```python
from build123d import *

# Parameters (mm, degrees)
SKETCH_W           = 37
SKETCH_H           = 51.5
PAD_DEPTH          = 25
SKETCH001_W        = 31
SKETCH001_H        = 45.5
POCKET_DEPTH       = 22
SKETCH002_W        = 31.0000008352
SKETCH002_H        = 3
POCKET001_DEPTH    = 22
SKETCH003_R        = 2
POCKET002_DEPTH    = 5
SKETCH004_R        = 3
POCKET003_DEPTH    = 1
SKETCH005_W        = 4
SKETCH005_H        = 3
PAD001_DEPTH       = 22
PAD001_FACE12_W    = 45.5
PAD001_FACE12_H    = 22
POCKET004_DEPTH    = 0.1
POCKET004_FACE17_W = 3.9999991648
POCKET004_FACE17_H = 22
POCKET005_DEPTH    = 0.1
POCKET005_FACE13_W = 31
POCKET005_FACE13_H = 22
POCKET006_DEPTH    = 0.1
POCKET006_FACE12_W = 45.5
POCKET006_FACE12_H = 22
POCKET007_DEPTH    = 0.1
POCKET007_FACE11_W = 4
POCKET007_FACE11_H = 22
POCKET008_DEPTH    = 0.1
POCKET008_FACE19_W = 0.1
POCKET008_FACE19_H = 22
POCKET009_DEPTH    = 0.1
POCKET009_FACE15_W = 0.1
POCKET009_FACE15_H = 22
POCKET010_DEPTH    = 0.1
POCKET010_FACE12_W = 0.1
POCKET010_FACE12_H = 22
POCKET011_DEPTH    = 0.1
POCKET011_FACE22_W = 0.1
POCKET011_FACE22_H = 22
POCKET012_DEPTH    = 0.1
POCKET012_FACE22_W = 45.7
POCKET012_FACE22_H = 22
POCKET013_DEPTH    = 1
POCKET013_FACE12_W = 45.7
POCKET013_FACE12_H = 22
POCKET014_DEPTH    = 1
POCKET014_FACE22_W = 33.2
POCKET014_FACE22_H = 22
POCKET015_DEPTH    = 1
POCKET015_FACE17_W = 5.0999991648
POCKET015_FACE17_H = 22
POCKET016_DEPTH    = 1
POCKET016_FACE11_W = 5.1
POCKET016_FACE11_H = 22
POCKET017_DEPTH    = 1
POCKET017_FACE3_W  = 51.5
POCKET017_FACE3_H  = 25
PAD002_DEPTH       = 1
PAD002_FACE2_W     = 51.5
PAD002_FACE2_H     = 25
PAD003_DEPTH       = 1
PAD003_FACE2_W     = 39
PAD003_FACE2_H     = 25
PAD004_DEPTH       = 1
PAD005_DEPTH       = 1
PAD006_DEPTH       = 5
PAD007_DEPTH       = 3
SKETCH006_W        = 22.9999991648
SKETCH006_H        = 3
PAD008_DEPTH       = 10


with BuildPart() as part:
    # Sketch → Pad (new body)
    with BuildSketch(Plane.XY):
        with Locations((-15.7498351648, -0.8188517965)):
            Rectangle(SKETCH_W, SKETCH_H)
    extrude(amount=PAD_DEPTH)

    # Sketch001 (on Face6 of Pad) → Pocket (cut)
    with BuildSketch(Plane.XY.offset(25)):
        with Locations((-15.7498351648, -0.8188517965)):
            Rectangle(SKETCH001_W, SKETCH001_H)
    extrude(amount=-POCKET_DEPTH, mode=Mode.SUBTRACT)

    # Sketch002 (on Face5 of Pocket) → Pocket001 (cut)
    with BuildSketch(Plane.XY.offset(25)):
        with Locations((-15.7498355824, -25.0688517965)):
            Rectangle(SKETCH002_W, SKETCH002_H)
    extrude(amount=-POCKET001_DEPTH, mode=Mode.SUBTRACT)

    # Sketch003 (on Face12 of Pocket001) → Pocket002 (cut)
    with BuildSketch(Plane.XY.offset(3)):
        with Locations((-15.5998351648, 16.2811482035)):
            Circle(SKETCH003_R)
        with Locations((-27.1998351648, -19.5188517965)):
            Circle(SKETCH003_R)
        with Locations((-4.2998351648, -19.5188517965)):
            Circle(SKETCH003_R)
    extrude(amount=-POCKET002_DEPTH, mode=Mode.SUBTRACT)

    # Sketch004 (on Face4 of Pocket002) → Pocket003 (cut)
    with BuildSketch(Plane(origin=(0, 0, 0), x_dir=(1, 0, 0), z_dir=(0, 0, -1))):
        with Locations((-27.199835, 19.518852)):
            Circle(SKETCH004_R)
        with Locations((-4.29979, 19.518393)):
            Circle(SKETCH004_R)
        with Locations((-15.599835, -16.281149)):
            Circle(SKETCH004_R)
    extrude(amount=-POCKET003_DEPTH, mode=Mode.SUBTRACT)

    # Sketch005 (on Face15 of Pocket003) → Pad001 (join)
    with BuildSketch(Plane.XY.offset(3)):
        with Locations((-29.249836, -25.0688517965)):
            Rectangle(SKETCH005_W, SKETCH005_H)
        with Locations((-2.2498351648, -25.0688517965)):
            Rectangle(SKETCH005_W, SKETCH005_H)
    extrude(amount=PAD001_DEPTH)

    # Pad001 Face12 → Pocket004 (cut)
    with BuildSketch(Plane(origin=(-31.2498351648, -0.8188517965, 14), x_dir=(0, -1, 0), z_dir=(1, 0, 0))):
        Rectangle(PAD001_FACE12_W, PAD001_FACE12_H)
    extrude(amount=-POCKET004_DEPTH, mode=Mode.SUBTRACT)

    # Pocket004 Face17 → Pocket005 (cut)
    with BuildSketch(Plane(origin=(-29.2498355824, -23.5688517965, 14), x_dir=(1, 0, 0), z_dir=(0, 1, 0))):
        Rectangle(POCKET004_FACE17_W, POCKET004_FACE17_H)
    extrude(amount=-POCKET005_DEPTH, mode=Mode.SUBTRACT)

    # Pocket005 Face13 → Pocket006 (cut)
    with BuildSketch(Plane(origin=(-15.7498351648, 21.9311482035, 14), x_dir=(-1, 0, 0), z_dir=(0, -1, 0))):
        Rectangle(POCKET005_FACE13_W, POCKET005_FACE13_H)
    extrude(amount=-POCKET006_DEPTH, mode=Mode.SUBTRACT)

    # Pocket006 Face12 → Pocket007 (cut)
    with BuildSketch(Plane(origin=(-0.2498351648, -0.8188517965, 14), x_dir=(0, 1, 0), z_dir=(-1, 0, 0))):
        Rectangle(POCKET006_FACE12_W, POCKET006_FACE12_H)
    extrude(amount=-POCKET007_DEPTH, mode=Mode.SUBTRACT)

    # Pocket007 Face11 → Pocket008 (cut)
    with BuildSketch(Plane(origin=(-2.2498351648, -23.5688517965, 14), x_dir=(1, 0, 0), z_dir=(0, 1, 0))):
        Rectangle(POCKET007_FACE11_W, POCKET007_FACE11_H)
    extrude(amount=-POCKET008_DEPTH, mode=Mode.SUBTRACT)

    # Pocket008 Face19 → Pocket009 (cut)
    with BuildSketch(Plane(origin=(-31.2998351648, 21.9311482035, 14), x_dir=(-1, 0, 0), z_dir=(0, -1, 0))):
        Rectangle(POCKET008_FACE19_W, POCKET008_FACE19_H)
    extrude(amount=-POCKET009_DEPTH, mode=Mode.SUBTRACT)

    # Pocket009 Face15 → Pocket010 (cut)
    with BuildSketch(Plane(origin=(-0.1998351648, 21.9311482035, 14), x_dir=(-1, 0, 0), z_dir=(0, -1, 0))):
        Rectangle(POCKET009_FACE15_W, POCKET009_FACE15_H)
    extrude(amount=-POCKET010_DEPTH, mode=Mode.SUBTRACT)

    # Pocket010 Face12 → Pocket011 (cut)
    with BuildSketch(Plane(origin=(-0.2498351648, -23.6188517965, 14), x_dir=(0, 1, 0), z_dir=(-1, 0, 0))):
        Rectangle(POCKET010_FACE12_W, POCKET010_FACE12_H)
    extrude(amount=-POCKET011_DEPTH, mode=Mode.SUBTRACT)

    # Pocket011 Face22 → Pocket012 (cut)
    with BuildSketch(Plane(origin=(-31.2498351648, -23.6188517965, 14), x_dir=(0, -1, 0), z_dir=(1, 0, 0))):
        Rectangle(POCKET011_FACE22_W, POCKET011_FACE22_H)
    extrude(amount=-POCKET012_DEPTH, mode=Mode.SUBTRACT)

    # Pocket012 Face22 → Pocket013 (cut)
    with BuildSketch(Plane(origin=(-31.3498351648, -0.8188517965, 14), x_dir=(0, -1, 0), z_dir=(1, 0, 0))):
        Rectangle(POCKET012_FACE22_W, POCKET012_FACE22_H)
    extrude(amount=-POCKET013_DEPTH, mode=Mode.SUBTRACT)

    # Pocket013 Face12 → Pocket014 (cut)
    with BuildSketch(Plane(origin=(-0.1498351648, -0.8188517965, 14), x_dir=(0, 1, 0), z_dir=(-1, 0, 0))):
        Rectangle(POCKET013_FACE12_W, POCKET013_FACE12_H)
    extrude(amount=-POCKET014_DEPTH, mode=Mode.SUBTRACT)

    # Pocket014 Face22 → Pocket015 (cut)
    with BuildSketch(Plane(origin=(-15.7498351648, 22.0311482035, 14), x_dir=(-1, 0, 0), z_dir=(0, -1, 0))):
        Rectangle(POCKET014_FACE22_W, POCKET014_FACE22_H)
    extrude(amount=-POCKET015_DEPTH, mode=Mode.SUBTRACT)

    # Pocket015 Face17 → Pocket016 (cut)
    with BuildSketch(Plane(origin=(-29.7998355824, -23.6688517965, 14), x_dir=(1, 0, 0), z_dir=(0, 1, 0))):
        Rectangle(POCKET015_FACE17_W, POCKET015_FACE17_H)
    extrude(amount=-POCKET016_DEPTH, mode=Mode.SUBTRACT)

    # Pocket016 Face11 → Pocket017 (cut)
    with BuildSketch(Plane(origin=(-1.6998351648, -23.6688517965, 14), x_dir=(1, 0, 0), z_dir=(0, 1, 0))):
        Rectangle(POCKET016_FACE11_W, POCKET016_FACE11_H)
    extrude(amount=-POCKET017_DEPTH, mode=Mode.SUBTRACT)

    # Pocket017 Face3 → Pad002 (add)
    with BuildSketch(Plane(origin=(2.7501648352, -0.8188517965, 12.5), x_dir=(0, -1, 0), z_dir=(1, 0, 0))):
        Rectangle(POCKET017_FACE3_W, POCKET017_FACE3_H)
    extrude(amount=PAD002_DEPTH)

    # Pad002 Face2 → Pad003 (add)
    with BuildSketch(Plane(origin=(-34.2498351648, -0.8188517965, 12.5), x_dir=(0, 1, 0), z_dir=(-1, 0, 0))):
        Rectangle(PAD002_FACE2_W, PAD002_FACE2_H)
    extrude(amount=PAD003_DEPTH)

    # Pad003 Face2 → Pad004 (add)
    with BuildSketch(Plane(origin=(-15.7498351648, 24.9311482035, 12.5), x_dir=(1, 0, 0), z_dir=(0, 1, 0))):
        Rectangle(PAD003_FACE2_W, PAD003_FACE2_H)
    extrude(amount=PAD004_DEPTH)

    # Pad004 Face2 → Pad005 (add)
    with BuildSketch(Plane(origin=(-15.7498347143, -26.5688517965, 10.8816629908), x_dir=(-1, 0, 0), z_dir=(0, -1, 0))):
        Polygon((19.5000004505, 10.8816629908), (-19.4999995495, 10.8816629908), (-19.4999995495, -14.1183370092), (-11.4999995495, -14.1183370092), (-11.4999995495, 7.8816629908), (11.5000012857, 7.8816629908), (11.5000012857, -14.1183370092), (19.5000004505, -14.1183370092), align=None)
    extrude(amount=PAD005_DEPTH)

    # Pad005 Face1 → Pad006 (add)
    with BuildSketch(Plane(origin=(-15.7498347143, -27.5688517965, 10.8816629908), x_dir=(-1, 0, 0), z_dir=(0, -1, 0))):
        Polygon((19.5000004505, 10.8816629908), (-19.4999995495, 10.8816629908), (-19.4999995495, -14.1183370092), (-11.4999995495, -14.1183370092), (-11.4999995495, 7.8816629908), (11.5000012857, 7.8816629908), (11.5000012857, -14.1183370092), (19.5000004505, -14.1183370092), align=None)
    extrude(amount=PAD006_DEPTH)

    # Pad006 Face3 → Pad007 (add)
    with BuildSketch(Plane(origin=(-15.7498347143, -32.5688517965, 10.8816629908), x_dir=(-1, 0, 0), z_dir=(0, -1, 0))):
        Polygon((19.5000004505, 10.8816629908), (-19.4999995495, 10.8816629908), (-19.4999995495, -14.1183370092), (-11.4999995495, -14.1183370092), (-11.4999995495, 7.8816629908), (11.5000012857, 7.8816629908), (11.5000012857, -14.1183370092), (19.5000004505, -14.1183370092), align=None)
    extrude(amount=PAD007_DEPTH)

    # Sketch006 (on Face23 of Pad007) → Pad008 (join)
    with BuildSketch(Plane.XY.offset(3)):
        with Locations((-15.7498355824, -34.0688517965)):
            Rectangle(SKETCH006_W, SKETCH006_H)
    extrude(amount=PAD008_DEPTH)


solid = part.part
```
Read the model definition and answer for the solid it produces. Units are mm, in the model's axes. A direction names the side the tool comes from. Give positions to 0.01 mm unless a question says otherwise; leave off trailing zeros. Write each loop counter-clockwise with the first axis right and the second up, starting at its lowest first coordinate (ties: lowest second). Pieces come first, ordered by that corner, then holes. Notation, with made-up numbers: (17.5, 89) - (52.5, 89) arc R19 cw to (52.5, 98) - close; hole circle Ø6 at (-40, -23.75). An arc over 180 degrees is marked (long way). Write item = value, one per line. Start each with the question number.
Item 1: Find section D-D (y = -30). Give the vertices of the cut face in (x, z).
Item 2: A tool of negligible diameter and unlimited length cuts with its end or side. For faces 1 (the cylindrical face through (-24.34, -20.42, 0.49)), 2 (the flat face through (2, -5, 25)), 3 (the flat face through (-16, 23.031, 14)), from which of +Z, -Z, +X, -X, +Y, -Y can it reach the whole face along a straight path? Write none if from no direction.
Item 3: Find section B-B (y = 15). Give the vertices of the cut face in (x, z).
Item 4: Find section C-C (x = -22). Give the vertices of the cut face in (y, z).
Item 5: Find the intervals of material crossed by probe 1 along X at (y, z) = (17, 12.5); probe 2 along Y at (x, z) = (-3.5, 21); probe 3 along X at (y, z) = (-32.5, 20.5), in increasing order. Write a range as [from, to].
Item 6: Each of these flat-tipped pins is pushed along its axis until it touches: P1, Ø1.5, axis at x = -18, z = 14, coming from the -Y side; P2, Ø5, axis at x = -3.5, y = -13, coming from the +Z side; P3, Ø5, axis at x = -27.2, y = -19.52, coming from the -Z side. Where does it stop, or does it pass through?
Response:
q1.outline = (-35.25, 0) - (3.75, 0) - (3.75, 25) - (-4.25, 25) - (-4.25, 3) - (-27.25, 3) - (-27.25, 25) - (-35.25, 25) - close
q2.face_1 = -Z
q2.face_2 = +Z, +X, -X, +Y, -Y
q2.face_3 = +Z
q3.outline = (-35.25, 0) - (-18.31, 0) - (-18.31, 1) - (-17.14, 1) - (-17.14, 3) - (-32.35, 3) - (-32.35, 25) - (-35.25, 25) - close; (-14.06, 1) - (-12.89, 1) - (-12.89, 0) - (3.75, 0) - (3.75, 25) - (0.85, 25) - (0.85, 3) - (-14.06, 3) - close
q4.outline = (-35.57, 0) - (25.93, 0) - (25.93, 25) - (23.03, 25) - (23.03, 3) - (-32.57, 3) - (-32.57, 13) - (-35.57, 13) - close
q5.probe_1 = [-35.25, -32.35], [0.85, 3.75]
q5.probe_2 = [-35.57, -24.67], [23.03, 25.93]
q5.probe_3 = [-35.25, -27.25], [-4.25, 3.75]
q6.P1 = 23.03
q6.P2 = 3
q6.P3 = 1
